Here's how the part is built. I have some questions about the finished solid (model axes, mm). A direction names the side the tool comes from. Give positions to 0.01 mm unless a question says otherwise; leave off trailing zeros. Order: outer loops, then holes, each group sorted by start corner. A loop starts at its lowest first (then second) coordinate and runs counter-clockwise, first axis right, second up.
from build123d import *

# Parameters (mm, degrees)
SKETCH2_W           = 65
SKETCH2_H           = 65
BOSS_EXTRUDE1_DEPTH = 10
SKETCH3_W           = 65
SKETCH3_H           = 6
SKETCH3_W_2         = 6
SKETCH3_H_2         = 24
BOSS_EXTRUDE2_DEPTH = 17.5
SKETCH4_R           = 3.175
BOSS_EXTRUDE3_DEPTH = 10
SKETCH5_R           = 1.99
CUT_EXTRUDE1_DEPTH  = 63.706080247


with BuildPart() as part:
    # Sketch2 → Boss-Extrude1 (new body)
    with BuildSketch(Plane(origin=(0, 0, 0), x_dir=(1, 0, 0), z_dir=(0, 1, 0))):
        Rectangle(SKETCH2_W, SKETCH2_H)
    extrude(amount=-BOSS_EXTRUDE1_DEPTH)

    # Sketch3 → Boss-Extrude2 (add, symmetric)
    with BuildSketch(Plane(origin=(0, 0, 0), x_dir=(0, 0, -1), z_dir=(1, 0, 0))):
        with Locations((0, 27)):
            Rectangle(SKETCH3_W, SKETCH3_H)
        with Locations((29.5, 12)):
            Rectangle(SKETCH3_W_2, SKETCH3_H_2)
        with Locations((-29.5, 12)):
            Rectangle(SKETCH3_W_2, SKETCH3_H_2)
    extrude(amount=BOSS_EXTRUDE2_DEPTH, both=True)

    # Sketch4 → Boss-Extrude3 (add)
    # profile 1 of 2: a face of its own
    with BuildSketch(Plane(origin=(0, 0, 0), x_dir=(1, 0, 0), z_dir=(0, 1, 0))):
        Polygon((32.5, 44.45), (-32.5, 44.45), (-32.5, 32.5), (-17.5, 32.5), (-17.5, 26.5), (17.5, 26.5), (17.5, 32.5), (32.5, 32.5), align=None)
        with Locations(Location((0, 38.1, 0), (0, 0, 270))):
            Circle(SKETCH4_R, mode=Mode.SUBTRACT)
    # profile 2 of 2: a face of its own
    with BuildSketch(Plane(origin=(0, 0, 0), x_dir=(1, 0, 0), z_dir=(0, 1, 0))):
        Polygon((-17.5, -32.5), (-32.5, -32.5), (-32.5, -44.45), (32.5, -44.45), (32.5, -32.5), (17.5, -32.5), (17.5, -26.5), (-17.5, -26.5), align=None)
        with Locations(Location((0, -38.1, 0), (0, 0, 270))):
            Circle(SKETCH4_R, mode=Mode.SUBTRACT)
    extrude(amount=-BOSS_EXTRUDE3_DEPTH)

    # Sketch5 → Cut-Extrude1 (cut, through all)
    with BuildSketch(Plane(origin=(0, 0, 0), x_dir=(1, 0, 0), z_dir=(0, 1, 0))):
        with Locations(Location((-26.5, 18.5, 0), (0, 0, 270))):
            Circle(SKETCH5_R)
        with Locations(Location((26.5, 18.5, 0), (0, 0, 270))):
            Circle(SKETCH5_R)
        with Locations(Location((26.5, -18.5, 0), (0, 0, 270))):
            Circle(SKETCH5_R)
        with Locations(Location((-26.5, -18.5, 0), (0, 0, 270))):
            Circle(SKETCH5_R)
    extrude(amount=-CUT_EXTRUDE1_DEPTH, mode=Mode.SUBTRACT)


solid = part.part
Q1. If we section it at C-C on y = -6: List the corners of the cut face in (x, z) for me (3 decimals), plus the area to 3 significant figures.
Filled sheet:
outline: (-32.5, -44.45) - (32.5, -44.45) - (32.5, 44.45) - (-32.5, 44.45) - close; hole circle Ø3.98 at (-26.5, -18.5); hole circle Ø3.98 at (-26.5, 18.5); hole circle Ø6.35 at (0, -38.1); hole circle Ø6.35 at (0, 38.1); hole circle Ø3.98 at (26.5, -18.5); hole circle Ø3.98 at (26.5, 18.5)
area: 5,670 mm2
Q2. I'm going to push flat-ended pins straight in: P1, Ø1.5, axis at y = 5.5, z = -26.5, coming from the -X side; P2, Ø15, axis at y = 22, z = 6.5, coming from the +X side; P3, Ø10, axis at x = 0, z = -38.1, coming from the +Y side; P4, Ø3, axis at x = -26.5, z = -18.5, coming from the -Y side. Where does each tip first touch, or does it pass through?
Filled sheet:
P1: stops at x = -17.5
P2: stops at x = 17.5
P3: stops at y = 0
P4: passes through
Q3. If we section it at D-D on z = -18.5: List the corners of the cut face in (x, y) for me.
Filled sheet:
outline: (-32.5, -10) - (-28.49, -10) - (-28.49, 0) - (-32.5, 0) - close; (-24.51, -10) - (24.51, -10) - (24.51, 0) - (-24.51, 0) - close; (-17.5, 24) - (17.5, 24) - (17.5, 30) - (-17.5, 30) - close; (28.49, -10) - (32.5, -10) - (32.5, 0) - (28.49, 0) - close
Q4. For faces 1 (the face through (17.5, 25, 0)), 2 (the face through (0, 24, 0)), 3 (the face through (0.14, -4.93, -41.27)), which set-ups out of +Z, -Z, +X, -X, +Y, -Y let a thin tool reach every point of the face, with its end or its side?
Filled sheet:
face 1: +Z, -Z, +X, +Y
face 2: +X, -X
face 3: +Y, -Y
Q5. I need wall thicknesses on L1, parallel to Y at x = 12, z = -18.5; L2, parallel to Z at x = -6, y = 18.5; L3, parallel to X at y = -6, z = -38. Which ranges of each line are inside material? Lowest first, please.
Filled sheet:
L1: y = -10 to 0, 24 to 30
L2: z = -32.5 to -26.5, 26.5 to 32.5
L3: x = -32.5 to -3.17, 3.17 to 32.5
Q6. Thinking about a two-plate mould opening in Z: for faces 4 (the face through (-17.5, 25, 0)), 5 (the face through (0, 15, -32.5)), 6 (the face through (0, 15, 32.5)), 7 (the face through (24.735, -4.93, -17.582)), which applies, released by +Z, released by -Z, zero draft, split by the parting line, or undercut?
Filled sheet:
face 4: zero draft
face 5: released by -Z
face 6: released by +Z
face 7: undercut
Q7. If we section it at B-B on z = 38.1: List the corners of the cut face in (x, y) for me (3 decimals).
Filled sheet:
outline: (-32.5, -10) - (-3.175, -10) - (-3.175, 0) - (-32.5, 0) - close; (3.175, -10) - (32.5, -10) - (32.5, 0) - (3.175, 0) - close
Q8. If we section it at A-A on x = 0: List the corners of the cut face in (y, z) for me (3 decimals).
Filled sheet:
outline: (-10, -44.45) - (0, -44.45) - (0, -41.275) - (-10, -41.275) - close; (-10, -34.925) - (0, -34.925) - (0, -32.5) - (30, -32.5) - (30, 32.5) - (0, 32.5) - (0, 34.925) - (-10, 34.925) - close; (-10, 41.275) - (0, 41.275) - (0, 44.45) - (-10, 44.45) - close; hole (0, -26.5) - (24, -26.5) - (24, 26.5) - (0, 26.5) - close
